The drawing under review shows one solid part. Ordinate dimensions are in mm from its lowest x, y, z. Coordinates: 2 decimals unless noted, no trailing zeros. Order: outer loops, then holes, each group sorted by start corner. A loop starts at its lowest first (then second) coordinate and runs counter-clockwise, first axis right, second up.
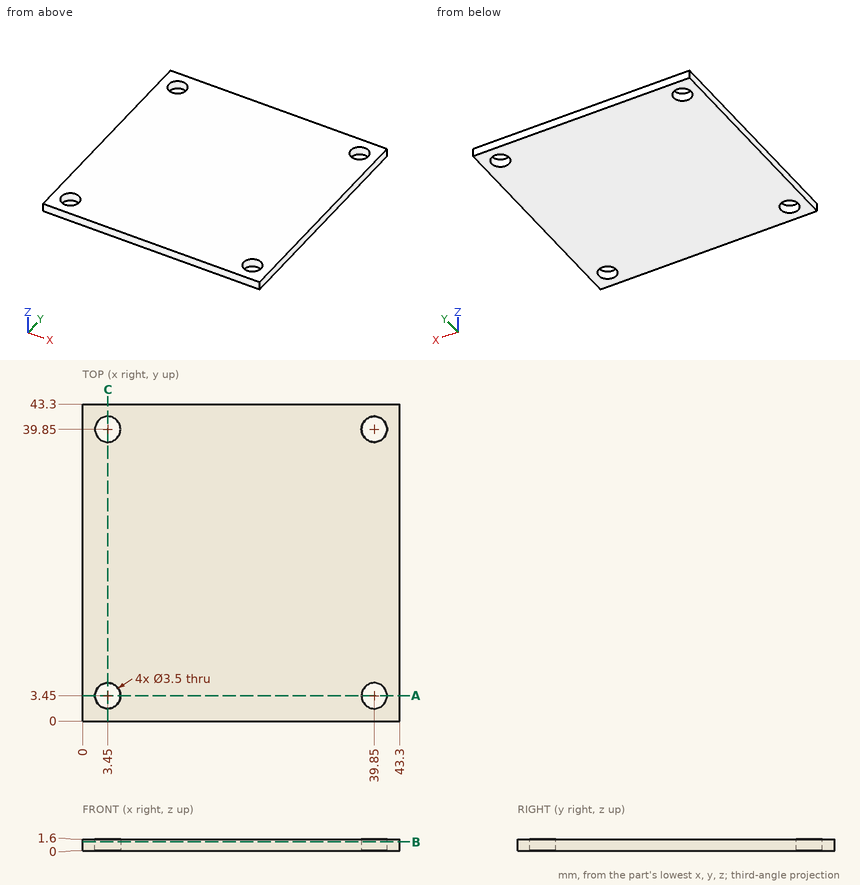
(1) Wall thickness on probe 1 along Y at (x, z) = (39.85, 0.9); probe 2 along Y at (x, z) = (3, 0.4): over which ranges is each line inside the solid? List them lowest first.
A:
probe 1: y = 0 to 1.7, 5.2 to 38.1, 41.6 to 43.3
probe 2: y = 0 to 1.76, 5.14 to 38.16, 41.54 to 43.3
(2) For pin 1 Ø5.5 at (x, y) = (3.45, 39.85) entering from +Z, flat-tipped, find the tip position at first contact; note if it passes through.
A:
pin 1: stops at z = 1.6
(3) We need section A-A, the plane y = 3.45. Write out the cut boundary in (x, z).
A:
outline: (0, 0) - (1.7, 0) - (1.7, 1.6) - (0, 1.6) - close; (5.2, 0) - (38.1, 0) - (38.1, 1.6) - (5.2, 1.6) - close; (41.6, 0) - (43.3, 0) - (43.3, 1.6) - (41.6, 1.6) - close
(4) We need section B-B, the plane z = 1.2. Write out the cut boundary in (x, y).
A:
outline: (0, 0) - (43.3, 0) - (43.3, 43.3) - (0, 43.3) - close; hole circle Ø3.5 at (3.45, 3.45); hole circle Ø3.5 at (3.45, 39.85); hole circle Ø3.5 at (39.85, 3.45); hole circle Ø3.5 at (39.85, 39.85)
